Check sheet for the modelled part. Datum: model origin and axes. Units: mm. A direction names the side the tool comes from. Round coordinates to 2 decimals unless told otherwise and drop trailing zeros. Write each loop counter-clockwise with the first axis right and the second up, starting at its lowest first coordinate (ties: lowest second). Pieces come first, ordered by that corner, then holes.
Item 1: Tool access check on faces 1 (the flat face through (12, 2, -7)), 2 (the flat face through (5.7, 0, -1.9)). Record the directions out of +Z, -Z, +X, -X, +Y, -Y that give a thin tool (end or side, any length) a straight path to the whole face; none if there is none.
Item 2: Material ranges on line 1 (X direction, y = 3.75, z = -10); line 2 (Z direction, x = 11.3, y = 4.5); line 3 (Y direction, x = 9.25, z = -10.75), recorded low to high.
Item 3: Go/stop test with flat-tipped pins: pin 1 Ø3 at (x, z) = (2, -10.5) entering from +Y; pin 2 Ø1.5 at (y, z) = (0, -7) entering from -X; pin 3 Ø3 at (y, z) = (7, -4) entering from -X. Record where each tip stops, or that it passes through.
Item 4: Cross-section at D-D on y = 4.5. Enter the section's corners in (x, z).
Item 5: Cross-section at C-C on x = 5. Enter the section's corners in (y, z).
Item 6: Release check for a two-part mould opening along Z. For faces 3 (the cylindrical face through (2.615, -1.993, -5.249)), 4 (the cylindrical face through (1.804, -1.268, -1.711)), 5 (the flat face through (9.5, 3, -2)), 6 (the conical face through (5, -1, -3)) record: +Z half, -Z half, draft (parallel to the pull), parting line (faces both ways), or undercut.
from build123d import *

# Parameters (mm, degrees)
RESSALTO_EXTRUS_O1_DEPTH = 12
FILETE1_R                = 6
FILETE2_R                = 6
ESBO_O3_R                = 2.5
CORTE_EXTRUS_O1_DEPTH    = 20.448650339
FILETE3_R                = 0.3
ESBO_O4_R                = 2.5
CORTE_EXTRUS_O2_DEPTH    = 19.013883535
CHANFRO2_SIZE            = 1.5


with BuildPart() as part:
    # Esboço2 → Ressalto-extrusão1 (new body)
    with BuildSketch(Plane.XY):
        Polygon((0, 0), (0, -2.5), (12, -2.5), (12, 9.5), (9.5, 9.5), (9.5, 0), align=None)
    extrude(amount=-RESSALTO_EXTRUS_O1_DEPTH)

    # Filete1
    filete1_edges = [part.edges().sort_by_distance(p)[0] for p in [
        (10.75, 9.5, 0),
        (10.75, 9.5, -12),
    ]]
    fillet(filete1_edges, radius=FILETE1_R - 0.0001)  # a hair under: the kernel refuses the full size

    # Filete2
    filete2_edges = [part.edges().sort_by_distance(p)[0] for p in [
        (0, -1.25, 0),
        (0, -1.25, -12),
    ]]
    fillet(filete2_edges, radius=FILETE2_R - 0.0001)  # a hair under: the kernel refuses the full size

    # Esboço3 → Corte-extrusão1 (cut, through all)
    with BuildSketch(Plane(origin=(0, 0, 0), x_dir=(1, 0, 0), z_dir=(0, 1, 0))):
        with Locations(Location((5, 6, 0), (0, 0, 180))):
            Circle(ESBO_O3_R)
    extrude(amount=-CORTE_EXTRUS_O1_DEPTH, mode=Mode.SUBTRACT)

    # Filete3
    filete3_edges = [part.edges().sort_by_distance(p)[0] for p in [
        (9.5, 0, -6),
    ]]
    fillet(filete3_edges, radius=FILETE3_R)

    # Esboço4 → Corte-extrusão2 (cut, through all)
    with BuildSketch(Plane.ZY.offset(-9.5)):
        with Locations(Location((-6, 4.5, 0), (0, 0, 270))):
            Circle(ESBO_O4_R)
    extrude(amount=-CORTE_EXTRUS_O2_DEPTH, mode=Mode.SUBTRACT)

    # Chanfro2
    chanfro2_edges = [part.edges().sort_by_distance(p)[0] for p in [
        (7.5, 0, -6),
        (9.5, 7, -6),
    ]]
    chamfer(chanfro2_edges, length=CHANFRO2_SIZE)


solid = part.part
Response values:
1. face 1: +Z, -Z, +X, +Y, -Y
1. face 2: +Z, -Z, -X, +Y
2. line 1: x = 9.5 to 12
2. line 2: z = -11.92 to -8.5, -3.5 to -0.08
2. line 3: y = -2.5 to 0
3. pin 1: stops at y = 0
3. pin 2: stops at x = 0.01
3. pin 3: stops at x = 9.5
4. outline: (9.5, -11.92) - (12, -11.92) - (12, -8.5) - (11, -8.5) - (9.5, -10) - close; (9.5, -2) - (11, -3.5) - (12, -3.5) - (12, -0.08) - (9.5, -0.08) - close
5. outline: (-2.5, -11.92) - (0, -11.92) - (0, -10) - (-1.5, -8.5) - (-2.5, -8.5) - close; (-2.5, -3.5) - (-1.5, -3.5) - (0, -2) - (0, -0.08) - (-2.5, -0.08) - close
6. face 3: undercut
6. face 4: +Z half
6. face 5: draft
6. face 6: undercut
